Part model, mm, in its own coordinate system. A direction names the side the tool comes from. Coordinates: 2 decimals unless noted, no trailing zeros. Loops run counter-clockwise (first coordinate to the right, second up) from the corner with the lowest first, then second, coordinate; pieces in that order, holes last. Notation, with made-up numbers: M -12,57.5 L 39,57.5 A26 ccw 39,81.5 Z; hole C 36,41.25 d5. An arc over 180 degrees is marked long. Use a Markdown table: item, result. Add a question column.
1) Tool access for faces 4 (the cylindrical face through (-1, 2, -24)), 5 (the flat face through (-50, 22.738, -1)), 6 (the flat face through (-27, 80, -3)): list every direction of +Z, -Z, +X, -X, +Y, -Y with a clear straight run to the whole face (end or side of a thin tool).
2) Band-saw the part on A-A (y = 43.21). List the corners of the cut face in (x, z), plus the area to 3 significant figures.
3) Band-saw the part on C-C (x = -78.5). List the corners of the cut face in (y, z), plus the area to 3 significant figures.
4) Band-saw the part on D-D (y = 108.5). List the corners of the cut face in (x, z), plus the area to 3 significant figures.
5) Pin check, flat tips, straight feed: pin 1 Ø5.5 at (x, z) = (-15, -31.12) entering from +Y; pin 2 Ø9 at (x, y) = (-78.5, 43.21) entering from -Z. Stop position of each tip, or through.
6) Wall check: probe 1 along Y at (x, z) = (-78.5, -2.2); probe 2 along X at (y, z) = (43, -1); probe 3 along X at (y, z) = (143, -2). Give the ranges that are in metal, low to high. Write a range as from..to.
7) Pull direction Y, two halves, no side cores. Call faces 1 (the flat face through (-93.5, 66.3, -2.6)), 2 (the cylindrical face through (-20.54, 96.77, -1.48)), 3 (the cylindrical face through (-92, 1.43, -24.16)): released by +Y, released by -Y, zero draft, split by the parting line, or undercut.
from build123d import *

# Parameters (mm, degrees)
F0_W     = 93.5
F0_H     = 153.21
F0_R     = 4
F0_R_2   = 2.5
F0_W_2   = 29.1728788614
F0_H_2   = 110.4717357084
F1_DEPTH = 3
F2_W     = 93.5
F2_H     = 5
F3_DEPTH = 46
F4_R     = 2.4
F5_DEPTH = 5
F6_W     = 3
F6_H     = 15
F7_DEPTH = 15
F9_DEPTH = 93.501
F10_R    = 4.99999


# Not quite as in the source:
# - a fillet or chamfer is up to 0.001 mm smaller than in the source, because OpenCascade refuses the exact size


with BuildPart() as f1:
    # F0 (on Top) → F1 (new body)
    with BuildSketch(Plane.XY):
        with Locations((-46.75, 76.605)):
            Rectangle(F0_W, F0_H)
        with Locations((-78.5, 43.21)):
            Circle(F0_R, mode=Mode.SUBTRACT)
        with Locations((-20, 43.21)):
            Circle(F0_R, mode=Mode.SUBTRACT)
        with Locations((-78.5, 99.21)):
            Circle(F0_R_2, mode=Mode.SUBTRACT)
        with Locations((-49.5864394307, 77.9741321458)):
            Rectangle(F0_W_2, F0_H_2, mode=Mode.SUBTRACT)
        with Locations((-78.5, 143.71)):
            Circle(F0_R_2, mode=Mode.SUBTRACT)
        with Locations((-20, 99.21)):
            Circle(F0_R_2, mode=Mode.SUBTRACT)
        with Locations((-20, 143.71)):
            Circle(F0_R_2, mode=Mode.SUBTRACT)
    extrude(amount=-F1_DEPTH)

    # F2 (on face) → F3 (join)
    with BuildSketch(Plane(origin=(0, 0, -3), x_dir=(1, 0, 0), z_dir=(0, 0, -1))):
        with Locations((-46.75, -2.5)):
            Rectangle(F2_W, F2_H)
    extrude(amount=F3_DEPTH)

    # F4 (on face) → F5 (cut, through all)
    with BuildSketch(Plane.XZ):
        with Locations((-15, -31.12)):
            Circle(F4_R)
    extrude(amount=-F5_DEPTH, mode=Mode.SUBTRACT)

    # F6 (on face) → F7 (join)
    with BuildSketch(Plane(origin=(0, 5, 0), x_dir=(-1, 0, 0), z_dir=(0, 1, 0))):
        with Locations((1.5, -10.5)):
            Rectangle(F6_W, F6_H)
        with Locations((92, -10.5)):
            Rectangle(F6_W, F6_H)
    extrude(amount=F7_DEPTH)

    # F8 (on face) → F9 (cut, through all)
    with BuildSketch(Plane(origin=(-93.5, 0, 0), x_dir=(0, -1, 0), z_dir=(-1, 0, 0))):
        Polygon((-5, -18), (-20, -3), (-20, -18), align=None)
    extrude(amount=-F9_DEPTH, mode=Mode.SUBTRACT)

    # F10 (radius 5 in the source; OpenCascade refuses exactly that, so slightly less here)
    f10_edges = [f1.edges().sort_by_distance(p)[0] for p in [
        (0, 153.21, -1.5),
        (-93.5, 153.21, -1.5),
        (0, 0, -24.5),
        (-93.5, 0, -24.5),
        (-64.172879, 133.21, -1.5),
        (-64.172879, 22.738264, -1.5),
        (-35, 22.738264, -1.5),
        (-35, 133.21, -1.5),
    ]]
    fillet(f10_edges, radius=F10_R)


solid = f1.part
Entries:
| question | item | result |
|---|---|---|
| 1 | face 4 | +Z, -Z, +X, -Y |
| 1 | face 5 | +Z, -Z |
| 1 | face 6 | -Z, +Y |
| 2 | outline | M -93.5,-3 L -82.5,-3 L -82.5,0 L -93.5,0 Z; M -74.5,-3 L -64.17,-3 L -64.17,0 L -74.5,0 Z; M -35,-3 L -24,-3 L -24,0 L -35,0 Z; M -16,-3 L 0,-3 L 0,0 L -16,0 Z |
| 2 | area | 145 mm2 |
| 3 | outline | M 0,-49 L 5,-49 L 5,-3 L 39.21,-3 L 39.21,0 L 0,0 Z; M 47.21,-3 L 96.71,-3 L 96.71,0 L 47.21,0 Z; M 101.71,-3 L 141.21,-3 L 141.21,0 L 101.71,0 Z; M 146.21,-3 L 153.21,-3 L 153.21,0 L 146.21,0 Z |
| 3 | area | 636 mm2 |
| 4 | outline | M -93.5,-3 L -64.17,-3 L -64.17,0 L -93.5,0 Z; M -35,-3 L 0,-3 L 0,0 L -35,0 Z |
| 4 | area | 193 mm2 |
| 5 | pin 1 | y = 5 |
| 5 | pin 2 | z = -3 |
| 6 | probe 1 | 0..39.21, 47.21..96.71, 101.71..141.21, 146.21..153.21 |
| 6 | probe 2 | -93.5..-82.49, -74.51..-64.17, -35..-23.99, -16.01..0 |
| 6 | probe 3 | -93.5..-80.9, -76.1..-22.4, -17.6..0 |
| 7 | face 1 | zero draft |
| 7 | face 2 | undercut |
| 7 | face 3 | released by -Y |
